Work out the finished part from the listing and answer in its coordinate system (mm). Coordinates: 2 decimals unless noted, no trailing zeros. Loops run counter-clockwise (first coordinate to the right, second up) from the corner with the lowest first, then second, coordinate; pieces in that order, holes last. Notation, with made-up numbers: (29, 11) -> (48, 11) arc R11 cw to (48, 20) -> close; hole circle Ø11 at (53.5, -10.5). An arc over 180 degrees is marked (long way). Use a Markdown table: item, result.
from build123d import *

# Parameters (mm, degrees)
OTHER_194_OUTLINE_R   = 1.5
OTHER_194_OUTLINE_R_2 = 2
OTHER_194_OUTLINE_R_3 = 7.05
OTHER_194_OUTLINE_R_4 = 13
OTHER_194_DEPTH       = 4
SKETCH_2_R            = 21.5
CUT_EXTRUDE_1_DEPTH   = 97.648848933


# Read off the part's stored shape, not the designer's step: the other step
with BuildPart() as part:
    # Other 194 outline → Other 194 (new body)
    with BuildSketch(Plane(origin=(0, 0, 0), x_dir=(1, 0, 0), z_dir=(0, 1, 0))):
        with BuildLine():
            ThreePointArc((-80.038961039, 12.639806795), (-89.998966964, -0.163883698), (-79.719334557, -12.712404162))
            Line((-79.719334557, -12.712404162), (23.954102093, -34.889386216))
            ThreePointArc((23.954102093, -34.889386216), (28.077901504, -33.940370837), (29.997141433, -30.169048806))
            Line((29.997141433, -30.169048806), (30.982276884, -1.048102596))
            ThreePointArc((30.982276884, -1.048102596), (19.596811299, 24.020095481), (-7.246753247, 30.141077741))
            Line((-7.246753247, 30.141077741), (-80.038961039, 12.639806795))
        make_face()
        with BuildLine():
            ThreePointArc((-62.228072273, -8.273007388), (-63.252931738, -7.483002306), (-63.281586626, -6.189316158))
            ThreePointArc((-63.281586626, -6.189316158), (-63.134274256, -5.851850099), (-62.995261901, -5.510881125))
            ThreePointArc((-62.995261901, -5.510881125), (-61.849651838, -4.581154117), (-60.461969326, -5.082304763))
            Line((-60.461969326, -5.082304763), (-59.605161669, -6.078992007))
            ThreePointArc((-59.605161669, -6.078992007), (-59.452788579, -7.822528522), (-61.056402543, -8.523641489))
            Line((-61.056402543, -8.523641489), (-62.228072273, -8.273007388))
        make_face(mode=Mode.SUBTRACT)
        with BuildLine():
            Line((-25.836688979, -16.057557417), (-42.41065304, -12.512189235))
            ThreePointArc((-42.41065304, -12.512189235), (-43.596867532, -11.052331075), (-42.424246953, -9.581531412))
            Line((-42.424246953, -9.581531412), (-24.221088321, -5.510705486))
            ThreePointArc((-24.221088321, -5.510705486), (-22.837996114, -5.908978844), (-22.426909172, -7.288316817))
            Line((-22.426909172, -7.288316817), (-24.056103742, -14.904510924))
            ThreePointArc((-24.056103742, -14.904510924), (-24.707592613, -15.849805447), (-25.836688979, -16.057557417))
        make_face(mode=Mode.SUBTRACT)
        with Locations((25, -30)):
            Circle(OTHER_194_OUTLINE_R, mode=Mode.SUBTRACT)
        with Locations((-18.384776311, -18.384776311)):
            Circle(OTHER_194_OUTLINE_R_2, mode=Mode.SUBTRACT)
        with Locations((-12.374368671, -12.374368671)):
            Circle(OTHER_194_OUTLINE_R_2, mode=Mode.SUBTRACT)
        with Locations((12.374368671, -12.374368671)):
            Circle(OTHER_194_OUTLINE_R_2, mode=Mode.SUBTRACT)
        with Locations((18.384776311, -18.384776311)):
            Circle(OTHER_194_OUTLINE_R_2, mode=Mode.SUBTRACT)
        with Locations((-77, 0)):
            Circle(OTHER_194_OUTLINE_R_3, mode=Mode.SUBTRACT)
        with BuildLine():
            ThreePointArc((-60.461969326, 5.082304763), (-61.849651838, 4.581154117), (-62.995261901, 5.510881125))
            ThreePointArc((-62.995261901, 5.510881125), (-63.134274256, 5.851850099), (-63.281586626, 6.189316158))
            ThreePointArc((-63.281586626, 6.189316158), (-63.252931738, 7.483002306), (-62.228072273, 8.273007388))
            Line((-62.228072273, 8.273007388), (-61.056402543, 8.523641489))
            ThreePointArc((-61.056402543, 8.523641489), (-59.452788579, 7.822528522), (-59.605161669, 6.078992007))
            Line((-59.605161669, 6.078992007), (-60.461969326, 5.082304763))
        make_face(mode=Mode.SUBTRACT)
        with Locations((-55.6, 0)):
            Circle(OTHER_194_OUTLINE_R_2, mode=Mode.SUBTRACT)
        with BuildLine():
            Line((-49, 4), (-49, -4))
            ThreePointArc((-49, -4), (-48, -5), (-49, -6))
            Line((-49, -6), (-52, -6))
            ThreePointArc((-52, -6), (-53, -5), (-52, -4))
            Line((-52, -4), (-52, 4))
            ThreePointArc((-52, 4), (-53, 5), (-52, 6))
            Line((-52, 6), (-49, 6))
            ThreePointArc((-49, 6), (-48, 5), (-49, 4))
        make_face(mode=Mode.SUBTRACT)
        with Locations((-45.4, 0)):
            Circle(OTHER_194_OUTLINE_R_2, mode=Mode.SUBTRACT)
        with BuildLine():
            Line((-39, -0.79505171), (-39, 0.79505171))
            ThreePointArc((-39, 0.79505171), (-38.437804637, 1.965744865), (-37.172636716, 2.258893669))
            Line((-37.172636716, 2.258893669), (-33.617473054, 1.463841959))
            ThreePointArc((-33.617473054, 1.463841959), (-32.444836338, 0), (-33.617473054, -1.463841959))
            Line((-33.617473054, -1.463841959), (-37.172636716, -2.258893669))
            ThreePointArc((-37.172636716, -2.258893669), (-38.437804637, -1.965744865), (-39, -0.79505171))
        make_face(mode=Mode.SUBTRACT)
        with BuildLine():
            Line((-24.221088321, 5.510705486), (-42.424246953, 9.581531412))
            ThreePointArc((-42.424246953, 9.581531412), (-43.596867532, 11.052331075), (-42.41065304, 12.512189235))
            Line((-42.41065304, 12.512189235), (-25.836688979, 16.057557417))
            ThreePointArc((-25.836688979, 16.057557417), (-24.707592613, 15.849805447), (-24.056103742, 14.904510924))
            Line((-24.056103742, 14.904510924), (-22.426909172, 7.288316817))
            ThreePointArc((-22.426909172, 7.288316817), (-22.837996114, 5.908978844), (-24.221088321, 5.510705486))
        make_face(mode=Mode.SUBTRACT)
        Circle(OTHER_194_OUTLINE_R_4, mode=Mode.SUBTRACT)
        with Locations((-12.374368671, 12.374368671)):
            Circle(OTHER_194_OUTLINE_R_2, mode=Mode.SUBTRACT)
        with Locations((12.374368671, 12.374368671)):
            Circle(OTHER_194_OUTLINE_R_2, mode=Mode.SUBTRACT)
        with Locations((-18.384776311, 18.384776311)):
            Circle(OTHER_194_OUTLINE_R_2, mode=Mode.SUBTRACT)
        with Locations((18.384776311, 18.384776311)):
            Circle(OTHER_194_OUTLINE_R_2, mode=Mode.SUBTRACT)
    extrude(amount=OTHER_194_DEPTH)

    # Sketch 2 → Cut-Extrude 1 (cut, through all)
    with BuildSketch(Plane(origin=(0, 4, 0), x_dir=(1, 0, 0), z_dir=(0, 1, 0))):
        with Locations(Location((0, 0, 0), (0, 0, 270))):
            Circle(SKETCH_2_R)
    extrude(amount=-CUT_EXTRUDE_1_DEPTH, mode=Mode.SUBTRACT)


solid = part.part
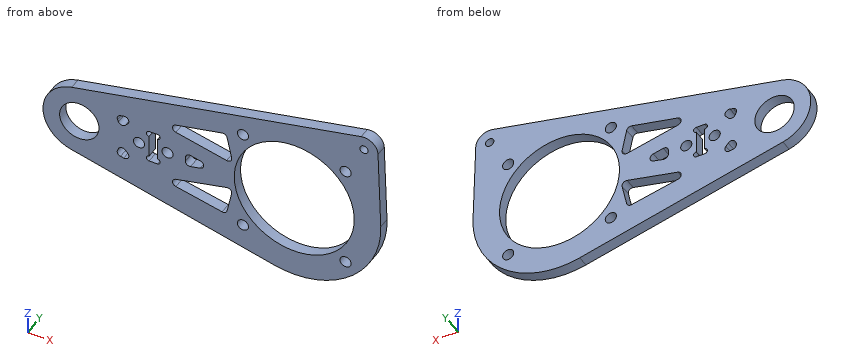
Q1. Section D-D on y = 0.8 is taken. State how many separate pieces and enclosed holes the cut face has, and give its area (3 significant figures).
Solved:
| item | result |
|---|---|
| separate pieces | 1 |
| enclosed holes | 15 |
| area | 3,360 mm² |
Q2. Given pin 1 Ø1.5 at (y, z) = (1.5, -3) entering from -X; pin 2 Ø3.5 at (x, z) = (-18.38, -18.38) entering from -Y; pin 3 Ø1.2 at (y, z) = (1.5, -1) entering from +X; pin 4 Ø1.5 at (x, y) = (-50, 3) entering from -Z, each flat-ended and moving along its own axis, determine where each tip first touches the part or whether it passes through.
Solved:
| item | result |
|---|---|
| pin 1 | x = -89.8 |
| pin 2 | through |
| pin 3 | x = 31 |
| pin 4 | z = -20.04 |
Q3. Consider line 1 (Z direction, x = -29.5, y = 2.25); line 2 (X direction, y = 1.5, z = -11); line 3 (Z direction, x = 25, y = 1.55). Determine where each line is inside the solid, lowest interval first. Write a range as [from, to].
Solved:
| item | result |
|---|---|
| line 1 | [-24.79, -15.27], [-6.69, 6.69], [15.27, 23.45] |
| line 2 | [-83.93, -43.6], [-23.22, -18.47], [18.47, 28.98] |
| line 3 | [-18.33, 28.5], [31.5, 35] |
Q4. Section A-A on x = -77 is taken. Determine the outline of the cut face in (y, z).
Solved:
| item | result |
|---|---|
| outline | (0, -13.37) -> (4, -13.37) -> (4, -7.05) -> (0, -7.05) -> close; (0, 7.05) -> (4, 7.05) -> (4, 13.29) -> (0, 13.29) -> close |
Q5. Section B-B on x = 2.5 is taken. Determine the outline of the cut face in (y, z), and give its area (3 significant figures).
Solved:
| item | result |
|---|---|
| outline | (0, -30.9) -> (4, -30.9) -> (4, -21.35) -> (0, -21.35) -> close; (0, 21.35) -> (4, 21.35) -> (4, 30.3) -> (0, 30.3) -> close |
| area | 74.0 mm² |
Q6. Section C-C on z = 23 is taken. Determine the outline of the cut face in (x, y).
Solved:
| item | result |
|---|---|
| outline | (-31.63, 0) -> (30.24, 0) -> (30.24, 4) -> (-31.63, 4) -> close |
